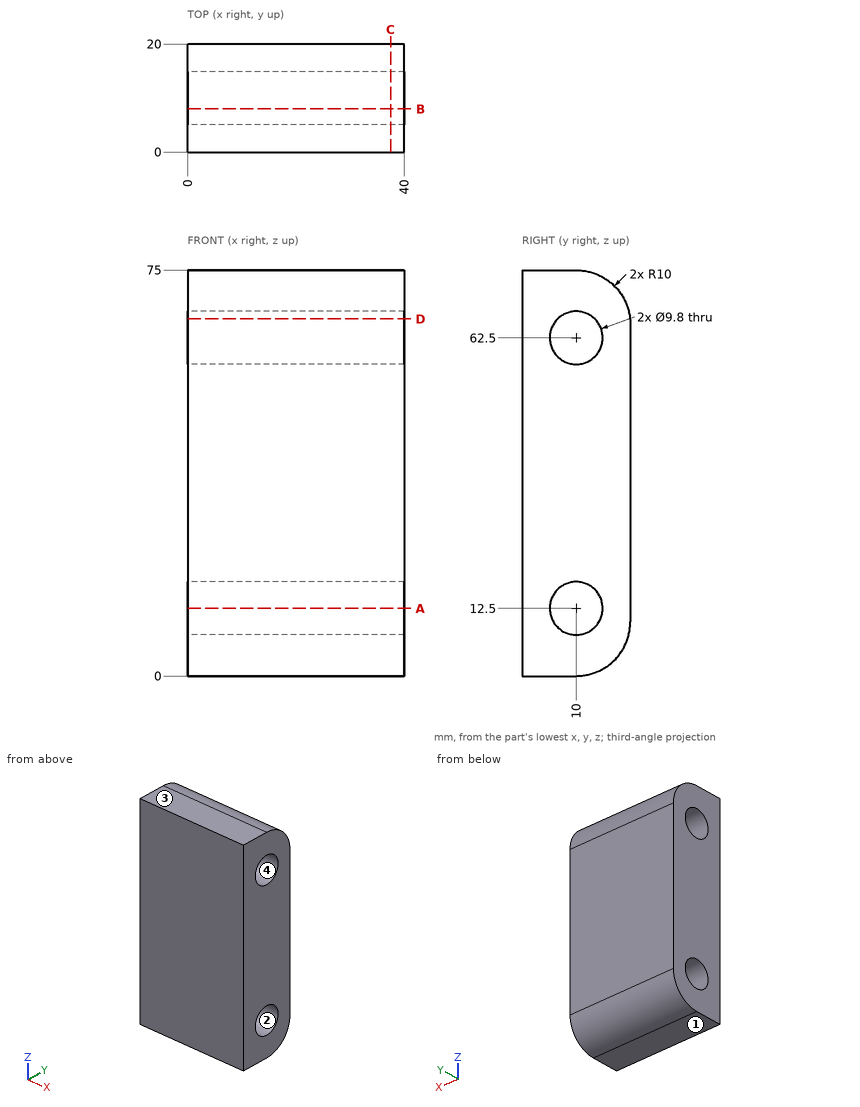
Could you check a few things on this drawing? It's one solid part, dimensions in mm from its lowest x, y, z. Coordinates: 2 decimals unless noted, no trailing zeros. Order: outer loops, then holes, each group sorted by start corner. A loop starts at its lowest first (then second) coordinate and runs counter-clockwise, first axis right, second up.
1) I need wall thicknesses on line 1 (Y direction, x = 10, z = 12.5); line 2 (Z direction, x = 24, y = 11.75); line 3 (Z direction, x = 12, y = 14.25). Which ranges of each line are inside material? Lowest first, please.
2) Will these pins go through, and if not, where does the flat tip stop? pin 1 (2 mm diameter, centred on y = 3, z = 9.5, fed in from -X); pin 2 (9 mm diameter, centred on y = 10, z = 62.5, fed in from -X).
3) Imagine slicing it at A-A on z = 12.5. List the corners of the cut face in (x, y) for me, and give its area (3 significant figures).
4) Imagine slicing it at D-D on z = 66. List the corners of the cut face in (x, y) for me.
5) We'd pull the mould along Z, two halves only. Please class the marked faces 1, 2, 3 and 4: +Z half, -Z half, draft (parallel to the pull), parting line (faces both ways), or undercut.
6) Imagine slicing it at C-C on x = 37.5. List the corners of the cut face in (y, z) for me.
7) Imagine slicing it at B-B on y = 8. List the corners of the cut face in (x, z) for me, and give its area (3 significant figures).
Response values:
1. line 1: y = 0 to 5.1, 14.9 to 20
1. line 2: z = 0.15 to 7.92, 17.08 to 57.92, 67.08 to 74.85
1. line 3: z = 0.95 to 10.06, 14.94 to 60.06, 64.94 to 74.05
2. pin 1: stops at x = 0
2. pin 2: passes through
3. outline: (0, 0) - (40, 0) - (40, 5.1) - (0, 5.1) - close; (0, 14.9) - (40, 14.9) - (40, 20) - (0, 20) - close
3. area: 408 mm2
4. outline: (0, 0) - (40, 0) - (40, 6.57) - (0, 6.57) - close; (0, 13.43) - (40, 13.43) - (40, 19.95) - (0, 19.95) - close
5. face 1: -Z half
5. face 2: undercut
5. face 3: +Z half
5. face 4: undercut
6. outline: (0, 0) - (10, 0) arc R10 ccw to (20, 10) - (20, 65) arc R10 ccw to (10, 75) - (0, 75) - close; hole circle Ø9.8 at (10, 12.5); hole circle Ø9.8 at (10, 62.5)
7. outline: (0, 0) - (40, 0) - (40, 8.03) - (0, 8.03) - close; (0, 16.97) - (40, 16.97) - (40, 58.03) - (0, 58.03) - close; (0, 66.97) - (40, 66.97) - (40, 75) - (0, 75) - close
7. area: 2,280 mm2
